Input: part model. Units: mm. Frame: model coordinates. Coordinates: 2 decimals unless noted, no trailing zeros. Loops run counter-clockwise (first coordinate to the right, second up) from the corner with the lowest first, then second, coordinate; pieces in that order, holes last.
(1) Line query: L1, parallel to X at y = 15, z = 1.6; L2, parallel to X at y = 20.5, z = 1.4; L3, parallel to X at y = 53, z = 2.4. Output: solid intervals per line, ascending.
(2) Section B-B, the plane y = 30.5. Return loops of the section in (x, z).
(3) Contact query for a flat-ended pin moving along its axis: P1, Ø1.5, axis at y = 46.5, z = 1, coming from the -X side. Output: stop coordinate, or through.
(4) Section A-A, the plane z = 2. Return loops of the section in (x, y), then the cut area to 3 significant figures.
```python
from build123d import *

# Parameters (mm, degrees)
SKETCH3_W           = 134.999984
SKETCH3_H           = 75.0000024
SKETCH3_R           = 1.5999968
SKETCH3_R_2         = 1.7499965
BOSS_EXTRUDE1_DEPTH = 3
FILLET1_R           = 8
FILLET2_R           = 2


with BuildPart() as part:
    # Sketch3 → Boss-Extrude1 (new body)
    # profile 1 of 4: a face of its own
    with BuildSketch(Plane.XY):
        with BuildLine():
            Line((10.0000054, 85.0000078), (-39.9999946, 85.0000078))
            Line((-39.9999946, 85.0000078), (-39.9999946, 78.0000078))
            ThreePointArc((-39.9999946, 78.0000078), (-37.878674256, 77.121328144), (-36.9999946, 75.0000078))
            ThreePointArc((-36.9999946, 75.0000078), (-37.878674256, 72.878687456), (-39.9999946, 72.0000078))
            Line((-39.9999946, 72.0000078), (-39.9999946, 67.0000078))
            Line((-39.9999946, 67.0000078), (-24.9999946, 67.0000078))
            Line((-24.9999946, 67.0000078), (-24.9999946, 28.0000054))
            Line((-24.9999946, 28.0000054), (-39.9999946, 28.0000054))
            Line((-39.9999946, 28.0000054), (-39.9999946, 23.0000054))
            ThreePointArc((-39.9999946, 23.0000054), (-37.878674256, 22.121325744), (-36.9999946, 20.0000054))
            ThreePointArc((-36.9999946, 20.0000054), (-37.878674256, 17.878685056), (-39.9999946, 17.0000054))
            Line((-39.9999946, 17.0000054), (-39.9999946, 10.0000054))
            Line((-39.9999946, 10.0000054), (10.0000054, 10.0000054))
            Line((10.0000054, 10.0000054), (10.0000054, 85.0000078))
        make_face()
    # profile 2 of 4: a face of its own
    with BuildSketch(Plane.XY):
        with BuildLine():
            Line((-39.9999946, 78.0000078), (-39.9999946, 85.0000078))
            Line((-39.9999946, 85.0000078), (-49.9999946, 85.0000078))
            Line((-49.9999946, 85.0000078), (-49.9999946, 67.0000078))
            Line((-49.9999946, 67.0000078), (-39.9999946, 67.0000078))
            Line((-39.9999946, 67.0000078), (-39.9999946, 72.0000078))
            ThreePointArc((-39.9999946, 72.0000078), (-42.9999946, 75.0000078), (-39.9999946, 78.0000078))
        make_face()
    # profile 3 of 4: a face of its own
    with BuildSketch(Plane.XY):
        with BuildLine():
            Line((-49.9999946, 10.0000054), (-39.9999946, 10.0000054))
            Line((-39.9999946, 10.0000054), (-39.9999946, 17.0000054))
            ThreePointArc((-39.9999946, 17.0000054), (-42.9999946, 20.0000054), (-39.9999946, 23.0000054))
            Line((-39.9999946, 23.0000054), (-39.9999946, 28.0000054))
            Line((-39.9999946, 28.0000054), (-49.9999946, 28.0000054))
            Line((-49.9999946, 28.0000054), (-49.9999946, 10.0000054))
        make_face()
    # profile 4 of 4: a face of its own
    with BuildSketch(Plane.XY):
        with Locations((77.4999974, 47.5000066)):
            Rectangle(SKETCH3_W, SKETCH3_H)
        with Locations((141.2748, 13.6144)):
            Circle(SKETCH3_R, mode=Mode.SUBTRACT)
        with Locations((141.0208, 49.2252)):
            Circle(SKETCH3_R_2, mode=Mode.SUBTRACT)
        with Locations((13.7725658, 81.3248056)):
            Circle(SKETCH3_R, mode=Mode.SUBTRACT)
        with Locations((13.6652, 13.843)):
            Circle(SKETCH3_R_2, mode=Mode.SUBTRACT)
    extrude(amount=BOSS_EXTRUDE1_DEPTH)

    # Fillet1
    fillet1_edges = [part.edges().sort_by_distance(p)[0] for p in [
        (144.9999894, 85.0000078, 1.5),
        (-49.9999946, 10.0000054, 1.5),
        (-49.9999946, 28.0000054, 1.5),
        (-24.9999946, 28.0000054, 1.5),
        (-24.9999946, 67.0000078, 1.5),
        (-49.9999946, 67.0000078, 1.5),
        (-49.9999946, 85.0000078, 1.5),
    ]]
    fillet(fillet1_edges, radius=FILLET1_R)

    # Fillet2
    fillet2_edges = [part.edges().sort_by_distance(p)[0] for p in [
        (144.9999894, 10.0000054, 1.5),
    ]]
    fillet(fillet2_edges, radius=FILLET2_R)


solid = part.part
```
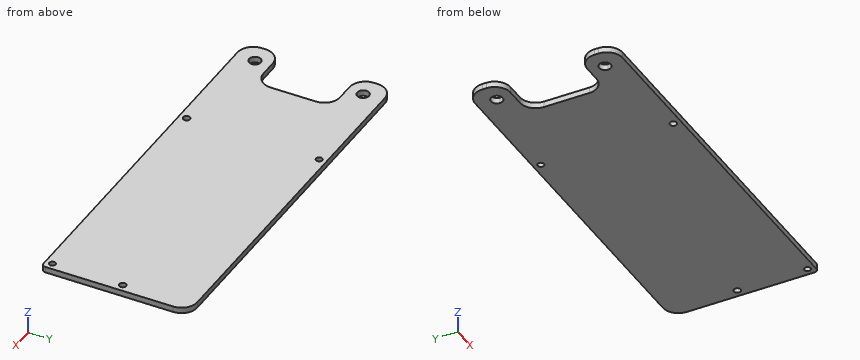
Report:
1. L1: x = -49.42 to 12.35, 14.98 to 140.47, 142.07 to 145
1. L2: x = -49.98 to -42.96, -37.04 to 145
1. L3: x = -25 to 145
2. outline: (-27.19, 0) - (145, 0) - (145, 3) - (-27.19, 3) - close
3. P1: stops at x = -25
4. outline: (-50, 18) arc R8 ccw to (-42, 10) - (143, 10) arc R2 ccw to (145, 12) - (145, 77) arc R8 ccw to (137, 85) - (-42, 85) arc R8 ccw to (-50, 77) - (-50, 75) arc R8 ccw to (-42, 67) - (-33, 67) arc R8 cw to (-25, 59) - (-25, 36) arc R8 cw to (-33, 28) - (-42, 28) arc R8 ccw to (-50, 20) - close; hole circle Ø6 at (-40, 20); hole circle Ø6 at (-40, 75); hole circle Ø3.5 at (13.67, 13.84); hole circle Ø3.2 at (13.77, 81.32); hole circle Ø3.5 at (141.02, 49.23); hole circle Ø3.2 at (141.27, 13.61)
4. area: 13,500 mm2
